Can you work these out from the model? Positions are in its coordinate system, mm. A direction names the side the tool comes from. Round coordinates to 2 decimals unless told otherwise and drop trailing zeros. Loops run counter-clockwise (first coordinate to the right, second up) from the corner with the lowest first, then second, coordinate; pieces in that order, holes last.
(1) If I drill on line 1 along X through (y, z) = (3.5, 9); line 2 along Z through (x, y) = (9, -1.5); line 3 along X through (y, z) = (-1.5, 1.5), over which ranges is the centre line in solid material (lowest first)?
(2) I want a section at B-B on x = -2.5. Write out the boundary of the cut face in (y, z).
(3) I want a section at C-C on z = -10.5. Write out the boundary of the cut face in (x, y), plus the area to 3 significant figures.
(4) Thinking about a two-plate mould opening in Z: for faces 1 (the face through (9.274, -3.042, -3.705)), 2 (the face through (-26, 0, 0)), which applies, released by +Z, released by -Z, zero draft, split by the parting line, or undercut?
(5) I want a section at D-D on y = 4.5. Write out the boundary of the cut face in (x, z).
(6) I want a section at A-A on y = 2.25. Give the number of separate pieces and of enclosed holes in the cut face, plus the area to 3 significant figures.
(7) Which directions (+Z, -Z, +X, -X, +Y, -Y) give clear straight access to the entire face, cutting with the end or side of a thin tool? Please do faces 3 (the face through (-7.5, -3, 7)), 4 (the face through (-3.2, 3.54, -5.66)), 5 (the face through (-10.22, 3.04, -5.1)).
(8) Will these pins go through, and if not, where does the flat tip stop? pin 1 Ø5 at (y, z) = (3.5, 8.5) entering from -X; pin 2 Ø3.5 at (x, z) = (11, -4.5) entering from -Y; pin 3 Ø2 at (y, z) = (-2.5, -7) entering from +X.
Autodesk Inventor part; units mm, degrees
ref_plane "Work Plane1" through (0, 0, -12.5) normal (0, 0, 1) x (1, 0, 0)
ref_plane "YZ Plane" through (0, 0, 0) normal (1, 0, 0) x (0, 1, 0)
ref_plane "XZ Plane" through (0, 0, 0) normal (0, 1, 0) x (-1, 0, 0)
ref_plane "Work Plane1" through (0, 0, -12.5) normal (0, 0, 1) x (1, 0, 0)
sketch "Sketch1" plane through (0, 0, -12.5) normal (0, 0, 1) x (1, 0, 0)
  arc A0 (20, -6) -> (20, 6) centre (20, 0) ccw
  line L0 (20, 6) -> (-20, 6)
  arc A1 (-20, 6) -> (-20, -6) centre (-20, 0) ccw
  line L1 (-20, -6) -> (20, -6)
extrude "Extrusion12" add sketch "Sketch1" along normal blind 25
sketch "Sketch2" plane through (-20, -6, -12.5) normal (0, -1, 0) x (1, 0, 0)
  line L0 (31, 10.5207) -> (27.5, 7.0207)
  line L1 (34.5, 7.0207) -> (31, 10.5207)
  line L2 (34.5, 2.9793) -> (34.5, 7.0207)
  line L3 (31, 0.9585) -> (34.5, 2.9793)
  line L4 (27.5, 2.9793) -> (31, 0.9585)
  line L5 (27.5, 7.0207) -> (27.5, 2.9793)
extrude "Extrusion11" cut sketch "Sketch2" against normal blind 6 draft 0
sketch "Sketch3" plane through (-20, -6, -12.5) normal (0, -1, 0) x (1, 0, 0)
  line L0 (9, 10.5207) -> (5.5, 7.0207)
  line L1 (12.5, 7.0207) -> (9, 10.5207)
  line L2 (12.5, 2.9793) -> (12.5, 7.0207)
  line L3 (9, 0.9585) -> (12.5, 2.9793)
  line L4 (5.5, 2.9793) -> (9, 0.9585)
  line L5 (5.5, 7.0207) -> (5.5, 2.9793)
extrude "Extrusion10" cut sketch "Sketch3" against normal blind 6 draft 0
sketch "Sketch4" plane through (-20, -6, -12.5) normal (0, -1, 0) x (1, 0, 0)
  line L0 (5.5, 22.0207) -> (5.5, 17.9793)
  line L1 (8.4793, 25) -> (9.5207, 25)
  line L2 (9, 15.9585) -> (12.5, 17.9793)
  line L3 (8.4793, 25) -> (5.5, 22.0207)
  line L4 (12.5, 22.0207) -> (9.5207, 25)
  line L5 (5.5, 17.9793) -> (9, 15.9585)
  line L6 (12.5, 17.9793) -> (12.5, 22.0207)
extrude "Extrusion9" cut sketch "Sketch4" against normal blind 6 draft 0
sketch "Sketch5" plane through (-20, -6, -12.5) normal (0, -1, 0) x (1, 0, 0)
  line L0 (31, 15.9585) -> (34.5, 17.9793)
  line L1 (30.4793, 25) -> (27.5, 22.0207)
  line L2 (34.5, 22.0207) -> (31.5207, 25)
  line L3 (27.5, 17.9793) -> (31, 15.9585)
  line L4 (31.5207, 25) -> (30.4793, 25)
  line L5 (34.5, 17.9793) -> (34.5, 22.0207)
  line L6 (27.5, 22.0207) -> (27.5, 17.9793)
extrude "Extrusion8" cut sketch "Sketch5" against normal blind 6
sketch "Sketch6" plane through (0, 0, 0) normal (0, 1, 0) x (-1, 0, 0)
  arc A0 (-12.591, 9.091) -> (-9.409, 9.091) centre (-11, 7.5) ccw
  line L0 (-12.591, 9.091) -> (-11, 10.682)
  line L1 (-11, 10.682) -> (-9.409, 9.091)
extrude "Extrusion7" cut sketch "Sketch6" along normal blind 6 draft 0
sketch "Sketch7" plane through (-20, 6, -12.5) normal (0, 1, 0) x (1, 0, 0)
  line L0 (7.409, -21.591) -> (9, -23.182)
  arc A0 (10.591, -21.591) -> (7.409, -21.591) centre (9, -20) ccw
  line L1 (9, -23.182) -> (10.591, -21.591)
extrude "Extrusion6" cut sketch "Sketch7" against normal blind 6
sketch "Sketch8" plane through (-20, 6, -12.5) normal (0, 1, 0) x (1, 0, 0)
  arc A0 (32.591, -6.591) -> (29.409, -6.591) centre (31, -5) ccw
  line L0 (31, -8.182) -> (32.591, -6.591)
  line L1 (29.409, -6.591) -> (31, -8.182)
extrude "Extrusion5" cut sketch "Sketch8" against normal blind 6
sketch "Sketch9" plane through (-20, 6, -12.5) normal (0, 1, 0) x (1, 0, 0)
  arc A0 (10.591, -6.591) -> (7.409, -6.591) centre (9, -5) ccw
  line L0 (9, -8.182) -> (10.591, -6.591)
  line L1 (7.409, -6.591) -> (9, -8.182)
extrude "Extrusion4" cut sketch "Sketch9" against normal blind 6
sketch "Sketch10" plane through (-20, 6, -12.5) normal (0, 1, 0) x (1, 0, 0)
  line L0 (20, -22.7528) -> (26.5, -16.2528)
  line L1 (13.5, -16.2528) -> (20, -22.7528)
  line L2 (13.5, -8.7472) -> (13.5, -16.2528)
  line L3 (20, -4.9944) -> (13.5, -8.7472)
  line L4 (26.5, -8.7472) -> (20, -4.9944)
  line L5 (26.5, -16.2528) -> (26.5, -8.7472)
extrude "Extrusion3" cut sketch "Sketch10" against normal blind 5 draft 0
sketch "Sketch11" plane through (-20, -6, -12.5) normal (0, -1, 0) x (1, 0, 0)
  line L0 (20, 23.8137) -> (14.3431, 18.1569)
  line L1 (25.6569, 18.1569) -> (20, 23.8137)
  arc A0 (14.3431, 18.1569) -> (25.6569, 18.1569) centre (20, 12.5) ccw
extrude "Extrusion2" cut sketch "Sketch11" against normal blind 2 draft 0
sketch "Sketch12" plane through (-20, 1, -12.5) normal (0, 1, 0) x (1, 0, 0)
  arc A0 (23.5355, -16.0355) -> (16.4645, -16.0355) centre (20, -12.5) ccw
  line L0 (20, -19.5711) -> (23.5355, -16.0355)
  line L1 (16.4645, -16.0355) -> (20, -19.5711)
extrude "Extrusion1" cut sketch "Sketch12" against normal blind 5
hole "Hole2" at (20, 0, 12.5) direction (0, 0, -1) diameter 6.5 depth 25
sketch "Sketch13" plane through (0, 0, 12.5) normal (0, 0, 1) x (1, 0, 0)
  point P0 (20, 0)
hole "Hole1" at (-20, 0, 12.5) direction (0, 0, -1) diameter 6.5 depth 25
sketch "Sketch14" plane through (0, 0, 12.5) normal (0, 0, 1) x (1, 0, 0)
  point P0 (-20, 0)
properties part number "Hopper Nut Trap" material "ASA Plastic"
Filled sheet:
1. line 1: x = -24.87 to -12.68, -9.32 to -1.25, 1.25 to 9.32, 12.68 to 24.87
1. line 2: z = -12.5 to -10.39, -3.98 to 4.61, 11.02 to 12.5
1. line 3: x = -25.81 to -22.88, -17.12 to -4.77, 4.77 to 17.12, 22.88 to 25.81
2. outline: (-6, -12.5) - (6, -12.5) - (6, -6.06) - (1, -6.06) - (1, -4.33) - (-4, -4.33) - (-4, -7.6) - (-6, -7.6) - close; (-6, 8.81) - (-4, 8.81) - (-4, 4.57) - (1, 4.57) - (1, 7.75) - (6, 7.75) - (6, 12.5) - (-6, 12.5) - close
3. outline: (-20, -6) - (-12.8, -6) - (-12.8, 0) - (-9.2, 0) - (-9.2, -6) - (9.2, -6) - (9.2, 0) - (12.8, 0) - (12.8, -6) - (20, -6) arc R6 ccw to (20, 6) - (-20, 6) arc R6 ccw to start; hole circle Ø6.5 at (-20, 0); hole circle Ø6.5 at (20, 0)
3. area: 483 mm2
4. face 1: undercut
4. face 2: zero draft
5. outline: (-23.97, -12.5) - (23.97, -12.5) - (23.97, 12.5) - (-23.97, 12.5) - close; hole (-12.59, -5.91) arc R2.25 ccw (long way) to (-9.41, -5.91) - (-11, -4.32) - close; hole (-12.59, 9.09) arc R2.25 ccw (long way) to (-9.41, 9.09) - (-11, 10.68) - close; hole (-6.5, -3.75) - (0, -7.51) - (6.5, -3.75) - (6.5, 3.75) - (0, 10.25) - (-6.5, 3.75) - close; hole (9.41, -5.91) arc R2.25 ccw (long way) to (12.59, -5.91) - (11, -4.32) - close; hole (9.41, 9.09) arc R2.25 ccw (long way) to (12.59, 9.09) - (11, 10.68) - close
6. separate pieces: 3
6. enclosed holes: 5
6. area: 811 mm2
7. face 3: -Y
7. face 4: +Y
7. face 5: +Y, -Y
8. pin 1: stops at x = -25.92
8. pin 2: stops at y = 0
8. pin 3: stops at x = 25.81
